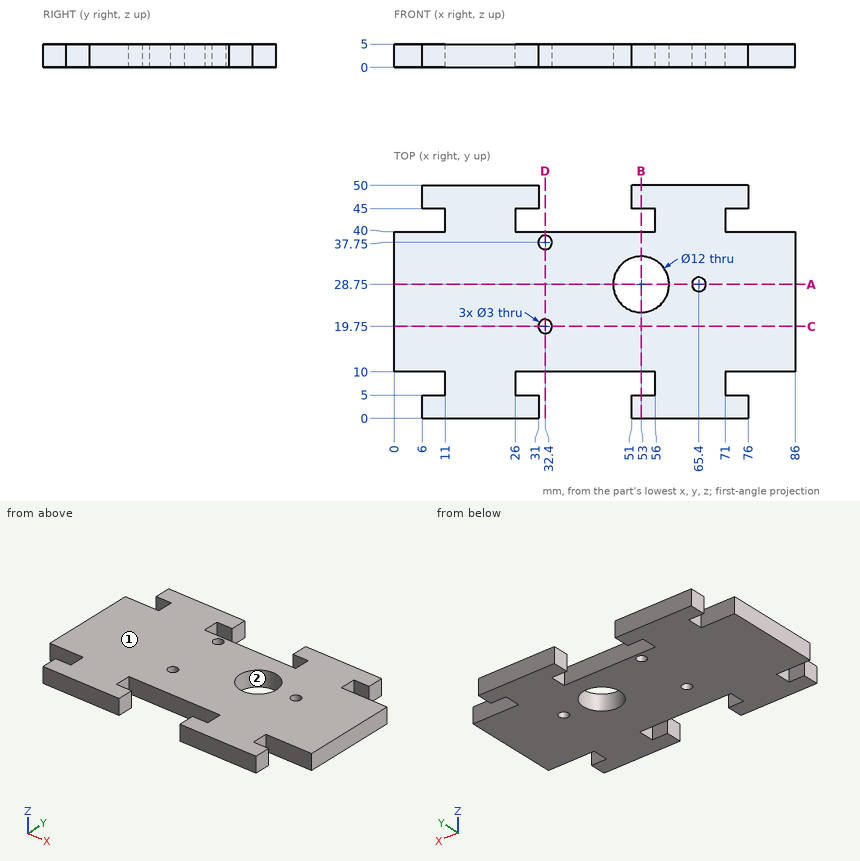
The figure shows three views and two pictorial views of one solid part (mm, origin at its lowest corner). Answer the questions. Coordinates: 2 decimals unless noted, no trailing zeros. Loops run counter-clockwise (first coordinate to the right, second up) from the corner with the lowest first, then second, coordinate; pieces in that order, holes last. Notation, with made-up numbers: (59.25, -30) -> (93.25, -30) arc R24 ccw to (93.25, -2) -> close; hole circle Ø11 at (71, 77). An arc over 180 degrees is marked (long way). Return JSON: item names as keys, results as strings. Group by question number.
(1) Find the intervals of material crossed by probe 1 along Y at (x, z) = (32.4, 1.1); probe 2 along Y at (x, z) = (74.5, 0.7); probe 3 along X at (y, z) = (27.5, 1.5), in increasing order. Write a range as from..to.
(2) Determine the mould class of the marked faces 1 and 2 for opening direction Y: released by +Y, released by -Y, zero draft, split by the parting line, or undercut.
(3) A cutting plane is placed at A-A on y = 28.75. Write down the section's boundary in (x, z).
(4) A cutting plane is placed at B-B on x = 53. Write down the section's boundary in (y, z), and give its area (3 significant figures).
(5) A cutting plane is placed at D-D on x = 32.4. Write down the section's boundary in (y, z).
(6) A cutting plane is placed at C-C on y = 19.75. Write down the section's boundary in (x, z).
(7) Given pin 1 Ø2.5 at (y, z) = (2.5, 2.5) entering from +X; pin 2 Ø2.5 at (x, y) = (32.4, 37.75) entering from +Z; pin 3 Ø1.5 at (y, z) = (6.5, 1.5) entering from -X; pin 4 Ø2.5 at (y, z) = (41.5, 1.5) entering from +X, each flat-ended and moving along its own axis, determine where each tip first touches the part or whether it passes through.
The answers:
{
 "1": {"probe 1": "y = 10..18.25, 21.25..36.25, 39.25..40", "probe 2": "y = 0..5, 10..40, 45..50", "probe 3": "x = 0..47.13, 58.87..64.57, 66.23..86"},
 "2": {"face 1": "zero draft", "face 2": "undercut"},
 "3": {"outline": "(0, 0) -> (47, 0) -> (47, 5) -> (0, 5) -> close; (59, 0) -> (63.9, 0) -> (63.9, 5) -> (59, 5) -> close; (66.9, 0) -> (86, 0) -> (86, 5) -> (66.9, 5) -> close"},
 "4": {"outline": "(0, 0) -> (5, 0) -> (5, 5) -> (0, 5) -> close; (10, 0) -> (22.75, 0) -> (22.75, 5) -> (10, 5) -> close; (34.75, 0) -> (40, 0) -> (40, 5) -> (34.75, 5) -> close; (45, 0) -> (50, 0) -> (50, 5) -> (45, 5) -> close", "area": "140 mm^2"},
 "5": {"outline": "(10, 0) -> (18.25, 0) -> (18.25, 5) -> (10, 5) -> close; (21.25, 0) -> (36.25, 0) -> (36.25, 5) -> (21.25, 5) -> close; (39.25, 0) -> (40, 0) -> (40, 5) -> (39.25, 5) -> close"},
 "6": {"outline": "(0, 0) -> (30.9, 0) -> (30.9, 5) -> (0, 5) -> close; (33.9, 0) -> (86, 0) -> (86, 5) -> (33.9, 5) -> close"},
 "7": {"pin 1": "stops at x = 76", "pin 2": "passes through", "pin 3": "stops at x = 11", "pin 4": "stops at x = 71"}
}
